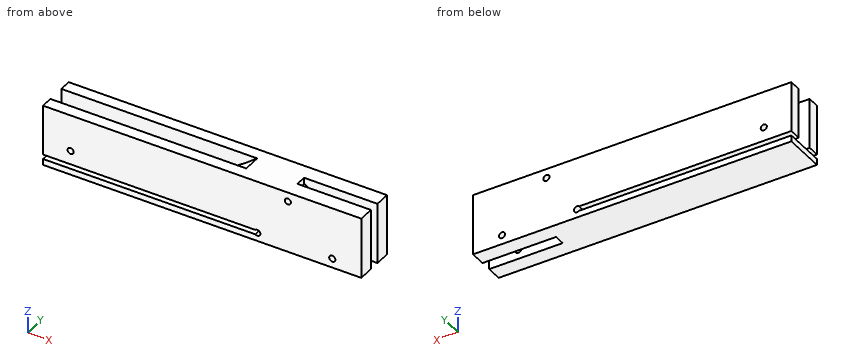
from build123d import *

# Parameters (mm, degrees)
F1_DEPTH  = 9.128125
F2_W      = 165.1
F2_H      = 31.75
F3_DEPTH  = 6.1293375
F4_W      = 165.1
F4_H      = 31.75
F5_DEPTH  = 6.1293375
F6_W      = 111.125
F6_H      = 2.38125
F7_DEPTH  = 21.3868
F8_R      = 1.5875
F9_DEPTH  = 21.3868
F11_DEPTH = 31.75


with BuildPart() as f1:
    # F0 (on Front) → F1 (new body)
    with BuildSketch(Plane.XZ):
        with BuildLine():
            Line((-57.15, -12.446), (-82.55, -12.446))
            Line((-82.55, -12.446), (-82.55, -15.621))
            Line((-82.55, -15.621), (82.55, -15.621))
            Line((82.55, -15.621), (82.55, 16.129))
            Line((82.55, 16.129), (19.05, 16.129))
            ThreePointArc((19.05, 16.129), (-16.6991764887, -4.4273626968), (-57.15, -12.446))
        make_face()
    extrude(amount=F1_DEPTH)

    # F2 (on face) → F3 (join)
    with BuildSketch(Plane.XZ.offset(9.128125)):
        with Locations((0, 0.254)):
            Rectangle(F2_W, F2_H)
    extrude(amount=F3_DEPTH)

    # F4 (on face) → F5 (join)
    with BuildSketch(Plane(origin=(0, 0, 0), x_dir=(-1, 0, 0), z_dir=(0, 1, 0))):
        with Locations((0, 0.254)):
            Rectangle(F4_W, F4_H)
    extrude(amount=F5_DEPTH)

    # F6 (on face) → F7 (cut, through all)
    with BuildSketch(Plane.XZ.offset(15.2574625)):
        with Locations((-26.9875, -11.255375)):
            Rectangle(F6_W, F6_H)
    extrude(amount=-F7_DEPTH, mode=Mode.SUBTRACT)

    # F8 (on face) → F9 (cut, through all)
    with BuildSketch(Plane.XZ.offset(15.2574625)):
        with Locations((-68.2625, -2.921)):
            Circle(F8_R)
        with Locations((28.575, -11.255375)):
            Circle(F8_R)
        with Locations((44.45, 11.3665)):
            Circle(F8_R)
        with Locations((67.46875, -10.8585)):
            Circle(F8_R)
    extrude(amount=-F9_DEPTH, mode=Mode.SUBTRACT)

    # F10 (on face) → F11 (cut, through all)
    with BuildSketch(Plane.XY.offset(16.129)):
        Polygon((82.55, -7.3421875), (82.55, -1.7859375), (44.45, -1.7859375), (44.45, -7.3421875), align=None)
    extrude(amount=-F11_DEPTH, mode=Mode.SUBTRACT)


solid = f1.part
Read the model definition and answer for the solid it produces. Units are mm, in the model's axes. Give positions to 0.01 mm unless a question says otherwise; leave off trailing zeros. Loops run counter-clockwise (first coordinate to the right, second up) from the corner with the lowest first, then second, coordinate; pieces in that order, holes last. Notation, with made-up numbers: (67, 48) - (103, 48) arc R18 ccw to (103, 62) - close; hole circle Ø1 at (-32, 84). An arc over 180 degrees is marked (long way). Answer as CSV lines item,"result". Start each with the question number.
1) Find section A-A (x = 56). Write down the section's boundary in (y, z).
2) Find section B-B (y = -12). State how many separate pieces and enclosed holes the cut face has, then the cut area to 3 significant figures.
3) Each of these flat-tipped pins is pushed along its axis until it touches: pin 1 Ø10 at (x, y) = (-42.5, -0.5) entering from +Z; pin 2 Ø1 at (y, z) = (-5, 14) entering from +X; pin 3 Ø3 at (x, z) = (67.47, -10.86) entering from +Y. Where does it stop, or does it pass through?
4) Find section D-D (x = -35). Write down the section's boundary in (y, z).
5) Find section C-C (z = 3.5). Write down the section's boundary in (x, y).
6) Straight lines are drawn through the part: L1, parallel to Y at x = -28, z = -6.5; L2, parallel to Y at x = 51, z = 3; L3, parallel to Z at x = 15.5, y = 5. For each, find the intervals that lie inside material, in ascending order. Write a range as from..to.
Findings below:
1,outline,"(-15.26, -15.62) - (-7.34, -15.62) - (-7.34, 16.13) - (-15.26, 16.13) - close; (-1.79, -15.62) - (6.13, -15.62) - (6.13, 16.13) - (-1.79, 16.13) - close"
2,separate pieces,"1"
2,enclosed holes,"3"
2,area,"4,950 mm^2"
3,pin 1,"z = 16.13"
3,pin 2,"x = 44.45"
3,pin 3,"through"
4,outline,"(-15.26, -15.62) - (6.13, -15.62) - (6.13, -12.45) - (-15.26, -12.45) - close; (-15.26, -10.06) - (6.13, -10.06) - (6.13, 16.13) - (0, 16.13) - (0, -9.76) - (-9.13, -9.76) - (-9.13, 16.13) - (-15.26, 16.13) - close"
5,outline,"(-82.55, -15.26) - (82.55, -15.26) - (82.55, -7.34) - (44.45, -7.34) - (44.45, -1.79) - (82.55, -1.79) - (82.55, 6.13) - (-82.55, 6.13) - (-82.55, 0) - (0.44, 0) - (0.44, -9.13) - (-82.55, -9.13) - close"
6,L1,"-15.26..-9.13, 0..6.13"
6,L2,"-15.26..-7.34, -1.79..6.13"
6,L3,"-15.62..-12.45, -10.06..16.13"
